```python
from build123d import *

# Parameters (mm, degrees)
SKETCH1_W           = 52.959
SKETCH1_H           = 9.525
BOSS_EXTRUDE3_DEPTH = 3.175
BOSS_EXTRUDE4_DEPTH = 9.525


with BuildPart() as part:
    # Sketch1 → Boss-Extrude3 (new body)
    with BuildSketch(Plane.XY):
        Rectangle(SKETCH1_W, SKETCH1_H)
    extrude(amount=BOSS_EXTRUDE3_DEPTH)

    # Sketch2 → Boss-Extrude4 (add)
    with BuildSketch(Plane.XY):
        Polygon((-26.4795, 4.7625), (-26.4795, -7.9375), (-23.3045, -7.9375), (-23.3045, 1.5875), (23.3045, 1.5875), (23.3045, -7.9375), (26.4795, -7.9375), (26.4795, 4.7625), align=None)
    extrude(amount=BOSS_EXTRUDE4_DEPTH)


solid = part.part
```
The listing builds one solid part. Answer for the finished solid, in the listing's coordinates (mm). A direction names the side the tool comes from. Give positions to 0.01 mm unless a question says otherwise; leave off trailing zeros. Order: outer loops, then holes, each group sorted by start corner. A loop starts at its lowest first (then second) coordinate and runs counter-clockwise, first axis right, second up. Notation, with made-up numbers: (33.25, -22.5) - (70.25, -22.5) arc R22 ccw to (70.25, 3.5) - close; hole circle Ø4 at (59, -16.75). An arc over 180 degrees is marked (long way). Answer in a Markdown table with one row per item. Add a question column.
Q1. Which of the six approach directions +Z, -Z, +X, -X, +Y, -Y give full straight-line access (tool end or side, diameter ignored) to faces 1 (the flat face through (26.48, -2, 5)), 2 (the flat face through (0, -4.762, 2)), 3 (the flat face through (23.304, -3, 6))?
Q2. Find the intervals of material crossed by line 1 along X through (y, z) = (-7, 2.5); line 2 along Y through (x, z) = (0.5, 8.5); line 3 along Z through (x, y) = (-4.5, -4.5) (3 decimals), in increasing order. Write a range as [from, to].
Q3. The part is cut by section D-D (z = 7). Determine the outline of the cut face in (x, y), then the cut area to 3 significant figures.
Q4. Given P1, Ø3, axis at x = 5.5, y = -1.5, coming from the +Z side (3 decimals); P2, Ø6, axis at x = 15, y = 0.5, coming from the -Z side; P3, Ø1, axis at x = -11.5, z = 5.5, coming from the -Y side; P4, Ø4, axis at x = -3, z = 1.5, coming from the -Y side, each flat-ended and moving along its own axis, determine where each tip first touches the part or whether it passes through.
Q5. The part is cut by section B-B (z = 2.5). Determine the outline of the cut face in (x, y).
Q6. For a pull along X with two mould halves and no side action, classify faces 4 (the flat face through (-26.48, -2, 5)), 5 (the flat face through (0, -2, 3.175)), 6 (the flat face through (-25, -7.938, 5)) as released by +X, released by -X, zero draft, split by the parting line, or undercut.
Q7. The part is cut by section A-A (y = -5.5). Determine the outline of the cut face in (x, z) (1 decimal), then the cut area to 3 significant figures.
Q8. The part is cut by section C-C (x = -17). Determine the outline of the cut face in (y, z) (1 decimal).
Determined:
| question | item | result |
|---|---|---|
| 1 | face 1 | +Z, -Z, +X, +Y, -Y |
| 1 | face 2 | +Z, -Z, -Y |
| 1 | face 3 | +Z, -Y |
| 2 | line 1 | x = [-26.48, -23.3], [23.3, 26.48] |
| 2 | line 2 | y = [1.59, 4.76] |
| 2 | line 3 | z = [0, 3.175] |
| 3 | outline | (-26.48, -7.94) - (-23.3, -7.94) - (-23.3, 1.59) - (23.3, 1.59) - (23.3, -7.94) - (26.48, -7.94) - (26.48, 4.76) - (-26.48, 4.76) - close |
| 3 | area | 229 mm² |
| 4 | P1 | stops at z = 3.175 |
| 4 | P2 | stops at z = 0 |
| 4 | P3 | stops at y = 1.59 |
| 4 | P4 | stops at y = -4.76 |
| 5 | outline | (-26.48, -7.94) - (-23.3, -7.94) - (-23.3, -4.76) - (23.3, -4.76) - (23.3, -7.94) - (26.48, -7.94) - (26.48, 4.76) - (-26.48, 4.76) - close |
| 6 | face 4 | released by -X |
| 6 | face 5 | undercut |
| 6 | face 6 | zero draft |
| 7 | outline | (-26.5, 0) - (-23.3, 0) - (-23.3, 9.5) - (-26.5, 9.5) - close; (23.3, 0) - (26.5, 0) - (26.5, 9.5) - (23.3, 9.5) - close |
| 7 | area | 60.5 mm² |
| 8 | outline | (-4.8, 0) - (4.8, 0) - (4.8, 9.5) - (1.6, 9.5) - (1.6, 3.2) - (-4.8, 3.2) - close |
